Build history of the part. All positions in model axes, mm. Round coordinates to 2 decimals unless told otherwise and drop trailing zeros. Loops run counter-clockwise (first coordinate to the right, second up) from the corner with the lowest first, then second, coordinate; pieces in that order, holes last. Notation, with made-up numbers: (4, 17.25) - (51, 17.25) arc R9 cw to (51, 27.25) - close; hole circle Ø6 at (79, -25). An arc over 180 degrees is marked (long way). Use a Markdown table: item, result.
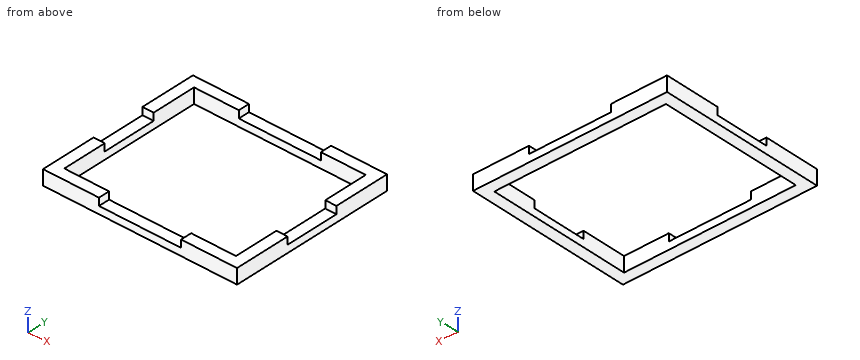
Autodesk Fusion 360 part; units mm, degrees
sketch "Sketch1" plane through (0, 0, 0) normal (0, 0, 1) x (1, 0, 0)
  line L0 (52, -44.5) -> (-52, -44.5)
  line L1 (-52, -44.5) -> (-52, 44.5)
  line L2 (-52, 44.5) -> (52, 44.5)
  line L3 (52, 44.5) -> (52, -44.5)
  line L4 (52, -44.5) -> (-52, 44.5) construction
  line L5 (-52, -44.5) -> (52, 44.5) construction
  dimension "d1" = 104
  dimension "d2" = 89
extrude "Extrude1" add sketch "Sketch1" along normal blind 8
sketch "Sketch4" plane through (0, 0, 8) normal (0, 0, 1) x (1, 0, 0)
  line L0 (46, -38.5) -> (-46, -38.5)
  line L1 (-46, -38.5) -> (-46, 38.5)
  line L2 (-46, 38.5) -> (46, 38.5)
  line L3 (46, 38.5) -> (46, -38.5)
  line L4 (46, -38.5) -> (-46, 38.5) construction
  line L5 (-46, -38.5) -> (46, 38.5) construction
  dimension "d5" = 77
  dimension "d6" = 92
extrude "Extrude2" cut sketch "Sketch4" against normal blind 8
sketch "Sketch5" plane through (0, 0, 8) normal (0, 0, 1) x (-1, 0, 0)
  line L0 (46, 38.5) -> (46, -38.5)
  line L1 (46, -38.5) -> (-46, -38.5)
  line L2 (-46, -38.5) -> (-46, 38.5)
  line L3 (-46, 38.5) -> (46, 38.5)
  line L4 (-52, -44.5) -> (52, -44.5)
  line L5 (52, -44.5) -> (52, 44.5)
  line L6 (52, 44.5) -> (-52, 44.5)
  line L7 (-52, 44.5) -> (-52, -44.5)
  line L8 (52, -14.5) -> (46, -14.5)
  line L9 (46, -14.5) -> (46, 14.5)
  line L10 (46, 14.5) -> (52, 14.5)
  line L11 (52, 14.5) -> (52, -14.5)
  dimension "d9" = 29
  dimension "d10" = 6
extrude "Extrude3" cut sketch "Sketch5" against normal blind 4 contours L0 L5 L8 L9 L10 L11
sketch "Sketch6" plane through (0, 0, 8) normal (0, 0, 1) x (-1, 0, 0)
  line L0 (46, 14.5) -> (52, 14.5)
  line L1 (52, 14.5) -> (52, 44.5)
  line L2 (52, 44.5) -> (-52, 44.5)
  line L3 (-52, 44.5) -> (-52, -44.5)
  line L4 (-52, -44.5) -> (52, -44.5)
  line L5 (52, -44.5) -> (52, -14.5)
  line L6 (52, -14.5) -> (46, -14.5)
  line L7 (46, -14.5) -> (46, -38.5)
  line L8 (46, -38.5) -> (-46, -38.5)
  line L9 (-46, -38.5) -> (-46, 38.5)
  line L10 (-46, 38.5) -> (46, 38.5)
  line L11 (46, 38.5) -> (46, 14.5)
  line L12 (-46, -14.5) -> (-52, -14.5)
  line L13 (-52, -14.5) -> (-52, 14.5)
  line L14 (-52, 14.5) -> (-46, 14.5)
  line L15 (-46, 14.5) -> (-46, -14.5)
  dimension "d13" = 29
  dimension "d14" = 6
extrude "Extrude4" cut sketch "Sketch6" against normal blind 4 contours L3 L9 L12 L13 L14 L15
sketch "Sketch7" plane through (0, 0, 8) normal (0, 0, 1) x (-1, 0, 0)
  line L0 (-46, -14.5) -> (-52, -14.5)
  line L1 (-52, -14.5) -> (-52, -44.5)
  line L2 (-52, -44.5) -> (52, -44.5)
  line L3 (52, -44.5) -> (52, -14.5)
  line L4 (52, -14.5) -> (46, -14.5)
  line L5 (46, -14.5) -> (46, -38.5)
  line L6 (46, -38.5) -> (-46, -38.5)
  line L7 (-46, -38.5) -> (-46, -14.5)
  line L8 (22, -44.5) -> (-22, -44.5)
  line L9 (-22, -44.5) -> (-22, -38.5)
  line L10 (-22, -38.5) -> (22, -38.5)
  line L11 (22, -38.5) -> (22, -44.5)
  dimension "d17" = 6
  dimension "d18" = 44
extrude "Extrude5" cut sketch "Sketch7" against normal blind 4 contours L2 L6 L8 L9 L10 L11
sketch "Sketch8" plane through (0, 0, 8) normal (0, 0, 1) x (-1, 0, 0)
  line L0 (-52, 14.5) -> (-46, 14.5)
  line L1 (-46, 14.5) -> (-46, 38.5)
  line L2 (-46, 38.5) -> (46, 38.5)
  line L3 (46, 38.5) -> (46, 14.5)
  line L4 (46, 14.5) -> (52, 14.5)
  line L5 (52, 14.5) -> (52, 44.5)
  line L6 (52, 44.5) -> (-52, 44.5)
  line L7 (-52, 44.5) -> (-52, 14.5)
  line L8 (22.0005, 38.5) -> (-21.9995, 38.5)
  line L9 (-21.9995, 38.5) -> (-21.9995, 44.5)
  line L10 (-21.9995, 44.5) -> (22.0005, 44.5)
  line L11 (22.0005, 44.5) -> (22.0005, 38.5)
  dimension "d21" = 44
  dimension "d22" = 6
extrude "Extrude6" cut sketch "Sketch8" against normal blind 4 contours L2 L6 L8 L9 L10 L11
Q1. Drop a flat-ended pin along its axis: pin 1 (1.8 mm diameter, centred on x = 7.5, y = 41, fed in from +Z). Give the stop position or say it passes through.
Results found:
| item | result |
|---|---|
| pin 1 | stops at z = 4 |
Q2. Probe line 1 (X direction, y = 24, z = 1); line 2 (Y direction, x = -35.5, z = 3.25); line 3 (X direction, y = 39.5, z = 4.5). List the from-to ranges inside material, lowest first.
Results found:
| item | result |
|---|---|
| line 1 | x = -52 to -46, 46 to 52 |
| line 2 | y = -44.5 to -38.5, 38.5 to 44.5 |
| line 3 | x = -52 to -22, 22 to 52 |
Q3. Cut at B-B, the plane x = -5. List the corners of the cut face in (y, z).
Results found:
| item | result |
|---|---|
| outline | (-44.5, 0) - (-38.5, 0) - (-38.5, 4) - (-44.5, 4) - close; (38.5, 0) - (44.5, 0) - (44.5, 4) - (38.5, 4) - close |
Q4. Cut at C-C, the plane y = -1. List the corners of the cut face in (x, z).
Results found:
| item | result |
|---|---|
| outline | (-52, 0) - (-46, 0) - (-46, 4) - (-52, 4) - close; (46, 0) - (52, 0) - (52, 4) - (46, 4) - close |
Q5. Cut at A-A, the plane z = 2.5. List the corners of the cut face in (x, y), plus the area to 3 significant figures.
Results found:
| item | result |
|---|---|
| outline | (-52, -44.5) - (52, -44.5) - (52, 44.5) - (-52, 44.5) - close; hole (-46, -38.5) - (46, -38.5) - (46, 38.5) - (-46, 38.5) - close |
| area | 2,170 mm2 |
